```python
from build123d import *
from OCP.BRepAlgoAPI import BRepAlgoAPI_Cut
from OCP.TopTools import TopTools_ListOfShape

# Parameters (mm, degrees)
SKETCH1_R                 = 0.9
BOSS_EXTRUDE1_DEPTH       = 8
SKETCH2_R                 = 7.75
SKETCH2_R_2               = 6
BOSS_EXTRUDE2_DEPTH       = 6.3
BOSS_EXTRUDE3_REACH       = 22.454
SKETCH4_W                 = 2.8
SKETCH4_H                 = 0.87750041
CUT_EXTRUDE1_REACH        = 27.201
CUT_EXTRUDE1_END_RADIUS   = 6
SKETCH3_R                 = 0.05
SHELL1_DEPTH              = 7
SHELL1_START              = 7
SHELL1_2_DEPTH            = 4.129175608
SHELL1_START_2            = 13.07082292
SHELL1_3_DEPTH            = 0.22917708
SHELL1_START_3            = 6.988561285
SHELL1_4_DEPTH            = 0.511438715
SKETCH2_2_R               = 6
CUT_EXTRUDE2_DEPTH        = 17.669133202
F_1_0MM_DOWEL_HOLE1_D     = 1
F_1_0MM_DOWEL_HOLE1_DEPTH = 3
F_1_0MM_DOWEL_HOLE1_TIP   = 0.30043031


with BuildPart() as part:
    # Sketch1 → Boss-Extrude1 (new body)
    with BuildSketch(Plane.XY):
        with BuildLine():
            Line((-7.5, -8.5), (7.5, -8.5))
            ThreePointArc((7.5, -8.5), (8.207106781, -8.207106781), (8.5, -7.5))
            Line((8.5, -7.5), (8.5, -1.9))
            Line((8.5, -1.9), (10, -1.9))
            ThreePointArc((10, -1.9), (11.9, 0), (10, 1.9))
            Line((10, 1.9), (8.5, 1.9))
            Line((8.5, 1.9), (8.5, 7.5))
            ThreePointArc((8.5, 7.5), (8.207106781, 8.207106781), (7.5, 8.5))
            Line((7.5, 8.5), (-7.5, 8.5))
            ThreePointArc((-7.5, 8.5), (-8.207106781, 8.207106781), (-8.5, 7.5))
            Line((-8.5, 7.5), (-8.5, 1.9))
            Line((-8.5, 1.9), (-10, 1.9))
            ThreePointArc((-10, 1.9), (-11.9, 0), (-10, -1.9))
            Line((-10, -1.9), (-8.5, -1.9))
            Line((-8.5, -1.9), (-8.5, -7.5))
            ThreePointArc((-8.5, -7.5), (-8.207106781, -8.207106781), (-7.5, -8.5))
        make_face()
        with Locations((-10, 0)):
            Circle(SKETCH1_R, mode=Mode.SUBTRACT)
        with Locations(Location((10, 0, 0), (0, 0, 180))):
            Circle(SKETCH1_R, mode=Mode.SUBTRACT)
    extrude(amount=BOSS_EXTRUDE1_DEPTH)

    # Sketch2 → Boss-Extrude2 (add)
    with BuildSketch(Plane(origin=(0, 0, 8), x_dir=(-1, 0, 0), z_dir=(0, 0, -1))):
        Circle(SKETCH2_R)
        Circle(SKETCH2_R_2, mode=Mode.SUBTRACT)
    extrude(amount=-BOSS_EXTRUDE2_DEPTH)

    # Sketch4 → Boss-Extrude3 (add, up to next)
    with BuildSketch(Plane.XY.offset(14.3), mode=Mode.PRIVATE) as boss_extrude3_sk1:
        with Locations((0, 8.061249795)):
            Rectangle(SKETCH4_W, SKETCH4_H)
    boss_extrude3_tool1 = extrude(boss_extrude3_sk1.sketch, amount=-BOSS_EXTRUDE3_REACH, mode=Mode.PRIVATE) - part.part
    add(boss_extrude3_tool1.solids().sort_by_distance((0, 8.06125, 14.3))[0])

    # Cut-Extrude1: up to this cylinder (the profile starts outside it)
    cut_extrude1_end = Plane(origin=(0, 0, 12.1), z_dir=(0, 0, -1)) * Cylinder(CUT_EXTRUDE1_END_RADIUS, 67.402, mode=Mode.PRIVATE)
    # Sketch3 → Cut-Extrude1 (cut, up to the surface)
    with BuildSketch(Plane(origin=(0, 8.5, 0), x_dir=(-1, 0, 0), z_dir=(0, 1, 0)), mode=Mode.PRIVATE) as cut_extrude1_sk1:
        with Locations(Location((0, 12.1, 0), (0, 0, 90))):
            Circle(SKETCH3_R)
    cut_extrude1_tool1 = extrude(cut_extrude1_sk1.sketch, amount=-CUT_EXTRUDE1_REACH, mode=Mode.PRIVATE) - cut_extrude1_end
    add(cut_extrude1_tool1.solids().sort_by_distance((0, 8.5, 12.1))[0], mode=Mode.SUBTRACT)


with BuildPart() as shell1_tool:
    # Shell1: read off the stored shape, not the designer's step
    # Shell1 outline → Shell1 (new body)
    with BuildSketch(Plane.XY):
        with BuildLine():
            Line((7.5, -0.9), (8.326679947, -0.9))
            ThreePointArc((8.326679947, -0.9), (8.1, 0), (8.326679947, 0.9))
            Line((8.326679947, 0.9), (7.5, 0.9))
            Line((7.5, 0.9), (7.5, 7.5))
            Line((7.5, 7.5), (-7.5, 7.5))
            Line((-7.5, 7.5), (-7.5, 0.9))
            Line((-7.5, 0.9), (-8.326679947, 0.9))
            ThreePointArc((-8.326679947, 0.9), (-8.1, 0), (-8.326679947, -0.9))
            Line((-8.326679947, -0.9), (-7.5, -0.9))
            Line((-7.5, -0.9), (-7.5, -7.5))
            Line((-7.5, -7.5), (7.5, -7.5))
            Line((7.5, -7.5), (7.5, -0.9))
        make_face()
    extrude(amount=SHELL1_DEPTH)


with BuildPart() as part_1:
    add(part.part)

    # Shell1: cut by shell1_tool, with a tolerance
    shell1_stock = TopTools_ListOfShape()
    shell1_stock.Append(part_1.part.wrapped)
    shell1_tools = TopTools_ListOfShape()
    shell1_tools.Append(shell1_tool.part.wrapped)
    shell1_cut = BRepAlgoAPI_Cut()
    shell1_cut.SetArguments(shell1_stock)
    shell1_cut.SetTools(shell1_tools)
    shell1_cut.SetFuzzyValue(0.00001)
    shell1_cut.Build()
    add(Compound.cast(shell1_cut.Shape()).solids(), mode=Mode.REPLACE)


with BuildPart() as shell1_2_tool:
    # Shell1 2 outline → Shell1 2 (new body)
    with BuildSketch(Plane.XY.offset(SHELL1_START)):
        with BuildLine():
            Line((0.4, 6.988562084), (0.4, 7.5))
            Line((0.4, 7.5), (-0.4, 7.5))
            Line((-0.4, 7.5), (-0.4, 6.988562084))
            ThreePointArc((-0.4, 6.988562084), (0, 7), (0.4, 6.988562084))
        make_face()
    extrude(amount=SHELL1_2_DEPTH)


with BuildPart() as part_2:
    add(part_1.part)

    # Shell1 2: cut by shell1_2_tool, with a tolerance
    shell1_2_stock = TopTools_ListOfShape()
    shell1_2_stock.Append(part_2.part.wrapped)
    shell1_2_tools = TopTools_ListOfShape()
    shell1_2_tools.Append(shell1_2_tool.part.wrapped)
    shell1_2_cut = BRepAlgoAPI_Cut()
    shell1_2_cut.SetArguments(shell1_2_stock)
    shell1_2_cut.SetTools(shell1_2_tools)
    shell1_2_cut.SetFuzzyValue(0.00001)
    shell1_2_cut.Build()
    add(Compound.cast(shell1_2_cut.Shape()).solids(), mode=Mode.REPLACE)


with BuildPart() as shell1_3_tool:
    # Shell1 3 outline → Shell1 3 (new body)
    with BuildSketch(Plane.XY.offset(SHELL1_START_2)):
        with BuildLine():
            Line((0.4, 6.988562084), (0.4, 7.5))
            Line((0.4, 7.5), (-0.4, 7.5))
            Line((-0.4, 7.5), (-0.4, 6.988562084))
            ThreePointArc((-0.4, 6.988562084), (0, 7), (0.4, 6.988562084))
        make_face()
    extrude(amount=SHELL1_3_DEPTH)


with BuildPart() as part_3:
    add(part_2.part)

    # Shell1 3: cut by shell1_3_tool, with a tolerance
    shell1_3_stock = TopTools_ListOfShape()
    shell1_3_stock.Append(part_3.part.wrapped)
    shell1_3_tools = TopTools_ListOfShape()
    shell1_3_tools.Append(shell1_3_tool.part.wrapped)
    shell1_3_cut = BRepAlgoAPI_Cut()
    shell1_3_cut.SetArguments(shell1_3_stock)
    shell1_3_cut.SetTools(shell1_3_tools)
    shell1_3_cut.SetFuzzyValue(0.00001)
    shell1_3_cut.Build()
    add(Compound.cast(shell1_3_cut.Shape()).solids(), mode=Mode.REPLACE)


with BuildPart() as shell1_4_tool:
    # Shell1 4 outline → Shell1 4 (new body)
    with BuildSketch(Plane(origin=(0, 0, 0), x_dir=(1, 0, 0), z_dir=(0, 1, 0)).offset(SHELL1_START_3)):
        with BuildLine():
            Line((-0.4, -11.129175608), (0.4, -11.129175608))
            ThreePointArc((0.4, -11.129175608), (0, -11.05), (-0.4, -11.129175608))
        make_face()
        with BuildLine():
            Line((0.4, -13.070824392), (-0.4, -13.070824392))
            ThreePointArc((-0.4, -13.070824392), (0, -13.15), (0.4, -13.070824392))
        make_face()
    extrude(amount=SHELL1_4_DEPTH)


with BuildPart() as part_4:
    add(part_3.part)


with BuildPart() as part_5:
    # Shell1 4: joined with shell1_4_tool
    add(part_4.part.fuse(shell1_4_tool.part, tol=0.00001))

    # Sketch2<2> → Cut-Extrude2 (cut, through all)
    with BuildSketch(Plane(origin=(0, 0, 8), x_dir=(-1, 0, 0), z_dir=(0, 0, -1))):
        Circle(SKETCH2_2_R)
    extrude(amount=CUT_EXTRUDE2_DEPTH, mode=Mode.SUBTRACT)

    # Ø1.0mm Dowel Hole1
    with Locations(Plane(origin=(0, 8.5, 12.1), x_dir=(0, 0, 1), z_dir=(0, 1, 0))):
        with Locations((0, 0)):
            Hole(F_1_0MM_DOWEL_HOLE1_D / 2, depth=F_1_0MM_DOWEL_HOLE1_DEPTH)
            with Locations((0, 0, -(F_1_0MM_DOWEL_HOLE1_DEPTH + F_1_0MM_DOWEL_HOLE1_TIP / 2))):  # 118° drill point
                Cone(0, F_1_0MM_DOWEL_HOLE1_D / 2, F_1_0MM_DOWEL_HOLE1_TIP, mode=Mode.SUBTRACT)


solid = part_5.part
```
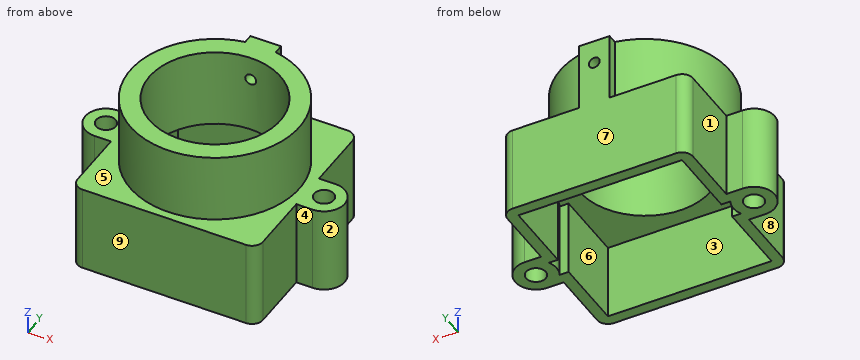
Read the model definition and answer for the solid it produces. Units are mm, in the model's axes. Face numbers are marked on the shaded views. A direction names the side the tool comes from. Coordinates: 2 decimals unless noted, no trailing zeros. Write each loop counter-clockwise with the first axis right and the second up, starting at its lowest first coordinate (ties: lowest second). Pieces come first, ordered by that corner, then holes. Notation, with made-up numbers: (20, 29.25) -> (78, 29.25) arc R24 ccw to (78, 67.25) -> close; hole circle Ø2 at (76, 66.5). An arc over 180 degrees is marked (long way). Answer as a JSON object with one key per item and string values.
Q1. Consider line 1 (Y direction, x = 0, z = 10.25); line 2 (Y direction, x = -10, z = 3); line 3 (Y direction, x = -3, z = 4.25). Determine where each line is inside the solid, lowest interval first. Write a range as [from, to].
The answers:
{"line 1": "y = [-7.75, -6], [6, 7], [7.5, 8.5]", "line 2": "y = [-1.9, -0.9], [0.9, 1.9]", "line 3": "y = [-8.5, -7.5], [7.5, 8.5]"}
Q2. Flat-ended cylindrical pins translate along their axes: pin 1 Ø6 at (y, z) = (-6, 3.5) entering from -X; pin 2 Ø5 at (y, z) = (-0.5, 12.5) entering from -X; pin 3 Ø4.5 at (y, z) = (4.5, 3) entering from +X. Find the tip coordinate at first contact, or state that the pin passes through.
The answers:
{"pin 1": "stops at x = -8.5", "pin 2": "stops at x = -7.75", "pin 3": "stops at x = 8.5"}
Q3. A tool of negligible diameter and unlimited length cuts with its end or side. For the marked faces 1, 2, 3, 4 and 5, from which of +Z, -Z, +X, -X, +Y, -Y can it reach the whole face along a straight path? Write none if from no direction.
The answers:
{"face 1": "+Z, -Z, -X, +Y", "face 2": "+Z, -Z, +X", "face 3": "-Z", "face 4": "+Z, -Z, +X, -Y", "face 5": "+Z"}
Q4. The part is cut by section D-D on x = 5.5. Give the vertices of the cut face in (y, z), then the cut area to 3 significant figures.
The answers:
{"outline": "(-8.5, 0) -> (-7.5, 0) -> (-7.5, 7) -> (-2.4, 7) -> (-2.4, 14.3) -> (-5.46, 14.3) -> (-5.46, 8) -> (-8.5, 8) -> close; (2.4, 7) -> (7.5, 7) -> (7.5, 0) -> (8.5, 0) -> (8.5, 8) -> (5.46, 8) -> (5.46, 14.3) -> (2.4, 14.3) -> close", "area": "64.8 mm2"}
Q5. The part is cut by section A-A on x = 0. Give the vertices of the cut face in (y, z).
The answers:
{"outline": "(-8.5, 0) -> (-7.5, 0) -> (-7.5, 7) -> (-6, 7) -> (-6, 14.3) -> (-7.75, 14.3) -> (-7.75, 8) -> (-8.5, 8) -> close; (6, 7) -> (7, 7) -> (7, 11.05) -> (7.5, 11.05) -> (7.5, 0) -> (8.5, 0) -> (8.5, 11.6) -> (6, 11.6) -> close; (6, 12.6) -> (8.5, 12.6) -> (8.5, 14.3) -> (6, 14.3) -> close; hole (7, 13.15) -> (7.5, 13.15) -> (7.5, 13.3) -> (7, 13.3) -> close"}
Q6. The part is cut by section C-C on z = 6.25. Give the number of separate pieces and of enclosed holes in the cut face, then the cut area to 3 significant figures.
The answers:
{"separate pieces": "1", "enclosed holes": "3", "area": "78.4 mm2"}
Q7. Determine the mould class of the marked faces 6, 7, 8 and 9 for opening direction Y: pulls with the +Y half, pulls with the -Y half, needs draft (parallel to the pull), parting line crosses it, or undercut.
The answers:
{"face 6": "undercut", "face 7": "pulls with the +Y half", "face 8": "needs draft", "face 9": "pulls with the -Y half"}
Q8. The part is cut by section B-B on y = 0. Give the vertices of the cut face in (x, z), then the cut area to 4 significant figures.
The answers:
{"outline": "(-11.9, 0) -> (-10.9, 0) -> (-10.9, 8) -> (-11.9, 8) -> close; (-9.1, 0) -> (-8.1, 0) -> (-8.1, 7) -> (-6, 7) -> (-6, 14.3) -> (-7.75, 14.3) -> (-7.75, 8) -> (-9.1, 8) -> close; (6, 7) -> (8.1, 7) -> (8.1, 0) -> (9.1, 0) -> (9.1, 8) -> (7.75, 8) -> (7.75, 14.3) -> (6, 14.3) -> close; (10.9, 0) -> (11.9, 0) -> (11.9, 8) -> (10.9, 8) -> close", "area": "58.25 mm2"}
